For this review, use the dimensioned drawing (mm, ordinates from the lowest corner) and the shaded views. A direction names the side the tool comes from. Give positions to 0.01 mm unless a question says otherwise; leave off trailing zeros. Loops run counter-clockwise (first coordinate to the right, second up) from the corner with the lowest first, then second, coordinate; pieces in that order, holes last. Notation, with made-up numbers: M 7,-23.5 L 38,-23.5 A13 ccw 38,-14.5 Z; hole C -40,6.5 d4. An arc over 180 degrees is marked long. Use a Markdown table: item, result. Add a question column.
(1) Add section B-B, the plane z = 5. Give the boundary of the cut face in (x, y) (1 decimal), then the cut area to 3 significant figures.
(2) Draft analysis for pull direction X (two halves, no side actions). For the marked faces 1 and 2, state which applies: pulls with the +X half, pulls with the -X half, needs draft (parallel to the pull), parting line crosses it, or undercut.
(3) Add section A-A, the plane y = 8. Give the boundary of the cut face in (x, z).
(4) For the marked faces 3 and 4, list the 3-axis set-ups (+Z, -Z, +X, -X, +Y, -Y) from which the entire face can be reached by the end or side of a thin tool; tool diameter is ignored.
(5) Insertion check: pin 1 Ø12 at (x, z) = (7.5, 12) entering from +Y (1 decimal); pin 2 Ø8 at (x, z) = (41.5, 22) entering from +Y (1 decimal); pin 3 Ø7 at (x, y) = (2.5, 23) entering from +Z (1 decimal); pin 4 Ø3.5 at (x, y) = (10, 22.5) entering from +Z. Each pin has a flat end and moves straight along its axis. Give the tip position at first contact, or say it passes through.
(6) Add section D-D, the plane z = 35.5. Give the boundary of the cut face in (x, y) (1 decimal).
(7) Add section C-C, the plane y = 17.75. Give the boundary of the cut face in (x, z).
(8) For probe 1 along Y at (x, z) = (38.5, 46.5) (1 decimal); probe 2 along X at (y, z) = (6, 54.5); probe 3 along Z at (x, y) = (49, 23.75), list the stretches that pass through material, from the lowest coordinate up.
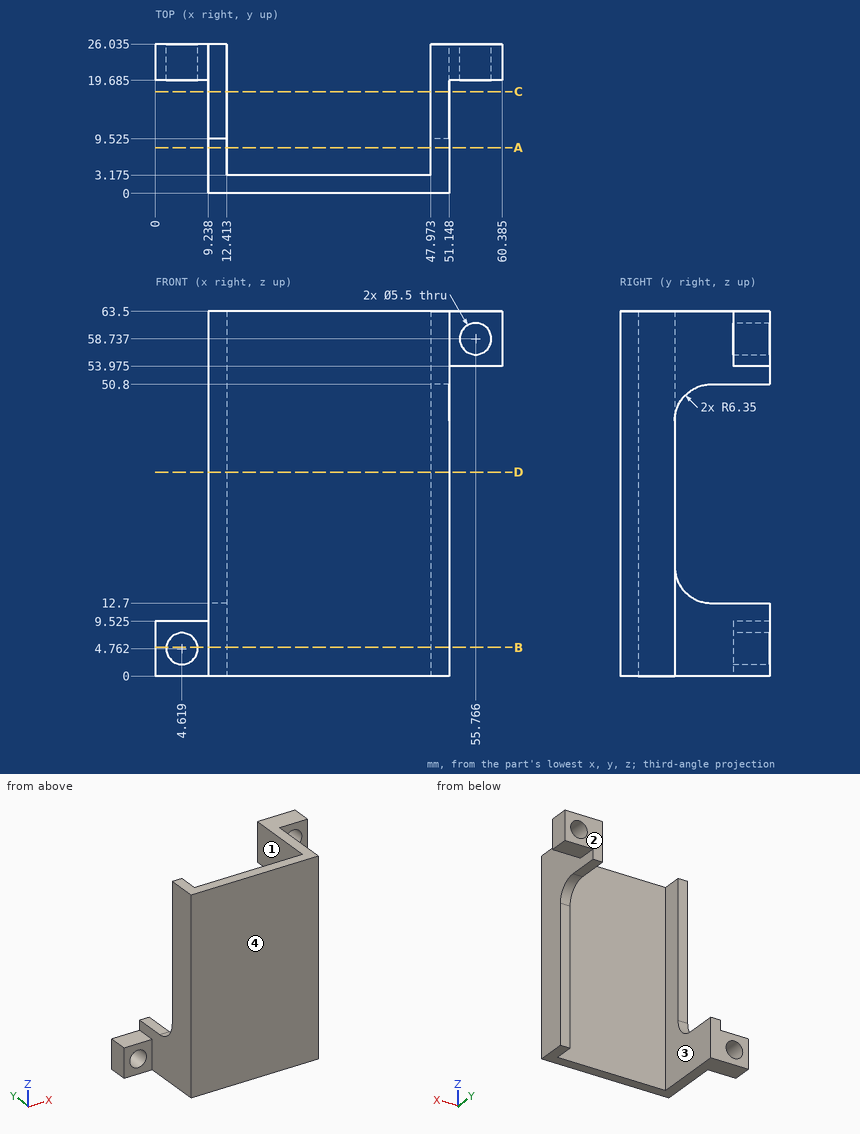
Established:
| question | item | result |
|---|---|---|
| 1 | outline | M 0,19.7 L 1.9,19.7 L 1.9,26 L 0,26 Z; M 7.4,19.7 L 9.2,19.7 L 9.2,0 L 51.1,0 L 51.1,9.5 L 48,9.5 L 48,3.2 L 12.4,3.2 L 12.4,26 L 7.4,26 Z |
| 1 | area | 250 mm^2 |
| 2 | face 1 | undercut |
| 2 | face 2 | needs draft |
| 3 | outline | M 9.24,0 L 12.41,0 L 12.41,63.5 L 9.24,63.5 Z; M 47.97,0 L 51.15,0 L 51.15,63.5 L 47.97,63.5 Z |
| 4 | face 3 | +Z, -Z, +Y |
| 4 | face 4 | +Z, -Z, +X, -X, -Y |
| 5 | pin 1 | y = 26 |
| 5 | pin 2 | y = 3.2 |
| 5 | pin 3 | z = 9.5 |
| 5 | pin 4 | z = 12.7 |
| 6 | outline | M 9.2,0 L 51.1,0 L 51.1,9.5 L 48,9.5 L 48,3.2 L 12.4,3.2 L 12.4,9.5 L 9.2,9.5 Z |
| 7 | outline | M 9.24,0 L 12.41,0 L 12.41,12.7 L 9.24,12.7 Z; M 47.97,50.8 L 51.15,50.8 L 51.15,63.5 L 47.97,63.5 Z |
| 8 | probe 1 | 0 to 3.2 |
| 8 | probe 2 | 9.24 to 12.41, 47.97 to 51.15 |
| 8 | probe 3 | 50.8 to 63.5 |
